Source: CAD feature listing. Evaluate the final solid. Frame: model axes, mm. A direction names the side the tool comes from. Give positions to 0.01 mm unless a question says otherwise; leave off trailing zeros. Loops run counter-clockwise (first coordinate to the right, second up) from the corner with the lowest first, then second, coordinate; pieces in that order, holes last.
from build123d import *

# Parameters (mm, degrees)
F0_W     = 50
F0_H     = 50
F1_DEPTH = 430
F2_W     = 20
F2_H     = 40
F3_DEPTH = 15
F4_W     = 20
F4_H     = 40
F5_DEPTH = 15


with BuildPart() as f1:
    # F0 (on Top) → F1 (new body)
    with BuildSketch(Plane.XY):
        with Locations((25, -25)):
            Rectangle(F0_W, F0_H)
    extrude(amount=F1_DEPTH)

    # F2 (on face) → F3 (cut)
    with BuildSketch(Plane.YZ.offset(50)):
        with Locations((-30, 400)):
            Rectangle(F2_W, F2_H)
        with Locations((-30, 330)):
            Rectangle(F2_W, F2_H)
        with Locations((-30, 260)):
            Rectangle(F2_W, F2_H)
        with Locations((-30, 190)):
            Rectangle(F2_W, F2_H)
        with Locations((-30, 120)):
            Rectangle(F2_W, F2_H)
    extrude(amount=-F3_DEPTH, mode=Mode.SUBTRACT)

    # F4 (on face) → F5 (cut)
    with BuildSketch(Plane(origin=(0, 0, 0), x_dir=(-1, 0, 0), z_dir=(0, 1, 0))):
        with Locations((-20, 400)):
            Rectangle(F4_W, F4_H)
        with Locations((-20, 330)):
            Rectangle(F4_W, F4_H)
        with Locations((-20, 260)):
            Rectangle(F4_W, F4_H)
        with Locations((-20, 190)):
            Rectangle(F4_W, F4_H)
        with Locations((-20, 120)):
            Rectangle(F4_W, F4_H)
    extrude(amount=-F5_DEPTH, mode=Mode.SUBTRACT)


solid = f1.part
1) Cut plane B-B (z = 126). Return loops of the section in (x, y), and give its area (3 significant figures).
Checks:
outline: (0, -50) - (50, -50) - (50, -40) - (35, -40) - (35, -20) - (50, -20) - (50, 0) - (30, 0) - (30, -15) - (10, -15) - (10, 0) - (0, 0) - close
area: 1,900 mm2
2) Ray query, probe 1 along Z at (x, y) = (45, -25); probe 2 along X at (y, z) = (-13, 384); probe 3 along Y at (x, z) = (35.5, 344). Return the intervals inside material, ascending.
Checks:
probe 1: z = 0 to 100, 140 to 170, 210 to 240, 280 to 310, 350 to 380, 420 to 430
probe 2: x = 0 to 10, 30 to 50
probe 3: y = -50 to -40, -20 to 0
3) Pull-direction query (Y, two-part tool) for faces 3 (the flat face through (20, -15, 400)), 4 (the flat face through (25, -25, 430)), 5 (the flat face through (43, -40, 330)); classes: released by +Y, released by -Y, zero draft, split by the parting line, or undercut.
Checks:
face 3: released by +Y
face 4: zero draft
face 5: undercut
4) Cut plane A-A (y = -6). Return loops of the section in (x, z), and give its area (3 significant figures).
Checks:
outline: (0, 0) - (50, 0) - (50, 430) - (0, 430) - close; hole (10, 100) - (30, 100) - (30, 140) - (10, 140) - close; hole (10, 170) - (30, 170) - (30, 210) - (10, 210) - close; hole (10, 240) - (30, 240) - (30, 280) - (10, 280) - close; hole (10, 310) - (30, 310) - (30, 350) - (10, 350) - close; hole (10, 380) - (30, 380) - (30, 420) - (10, 420) - close
area: 17,500 mm2
5) Cut plane C-C (x = 13.5). Return loops of the section in (y, z), and give its area (3 significant figures).
Checks:
outline: (-50, 0) - (0, 0) - (0, 100) - (-15, 100) - (-15, 140) - (0, 140) - (0, 170) - (-15, 170) - (-15, 210) - (0, 210) - (0, 240) - (-15, 240) - (-15, 280) - (0, 280) - (0, 310) - (-15, 310) - (-15, 350) - (0, 350) - (0, 380) - (-15, 380) - (-15, 420) - (0, 420) - (0, 430) - (-50, 430) - close
area: 18,500 mm2
6) Reachability of faces 1 (the flat face through (43, -20, 120)), 2 (the flat face through (20, -7, 350)) from +Z, -Z, +X, -X, +Y, -Y: full face, straight path, thin tool, end or side. Return the list, or none.
Checks:
face 1: +X
face 2: +Y
7) Contact query for a flat-ended pin moving along its axis: P1, Ø4, axis at y = -33.5, z = 130, coming from the +X side. Output: stop coordinate, or through.
Checks:
P1: stops at x = 35
